Can you work these out from the drawing? Everything is in mm from the part's minimum corner. Coordinates: 2 decimals unless noted, no trailing zeros. Loops run counter-clockwise (first coordinate to the right, second up) from the corner with the lowest first, then second, coordinate; pieces in that order, holes last. Notation, with made-up numbers: M -4.5,-29 L 10.5,-29 A22 ccw 10.5,8 Z; hole C -2.75,61 d2. An arc over 180 degrees is marked long. Write each question's results on one line, items separated by ' | '.
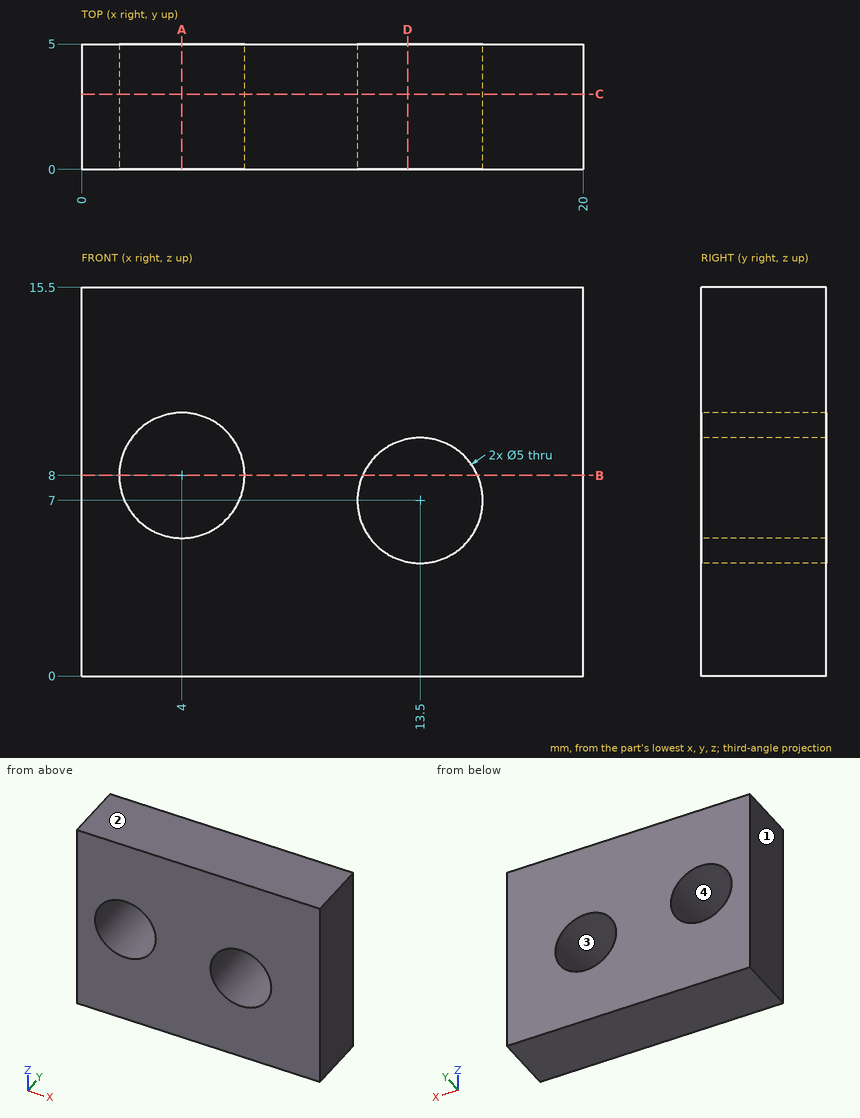
(1) Imagine slicing it at C-C, the plane y = 3. List the corners of the cut face in (x, z) for me.
Reported:
outline: M 0,0 L 20,0 L 20,15.5 L 0,15.5 Z; hole C 4,8 d5; hole C 13.5,7 d5
(2) Please list where these lines run through material, in increasing order: probe 1 along Z at (x, y) = (13.5, 3.7); probe 2 along Z at (x, y) = (4, 2.8); probe 3 along X at (y, z) = (1.5, 8.5). Write a range as from..to.
Reported:
probe 1: z = 0..4.5, 9.5..15.5 | probe 2: z = 0..5.5, 10.5..15.5 | probe 3: x = 0..1.55, 6.45..11.5, 15.5..20
(3) Will this pin go through, and if not, where does the flat tip stop? P1, Ø3, axis at x = 4, z = 8, coming from the +Y side.
Reported:
P1: passes through
(4) Imagine slicing it at B-B, the plane z = 8. List the corners of the cut face in (x, y) for me, and give its area (3 significant figures).
Reported:
outline: M 0,0 L 1.5,0 L 1.5,5 L 0,5 Z; M 6.5,0 L 11.21,0 L 11.21,5 L 6.5,5 Z; M 15.79,0 L 20,0 L 20,5 L 15.79,5 Z | area: 52.1 mm2
(5) Imagine slicing it at D-D, the plane x = 13. List the corners of the cut face in (y, z) for me, and give its area (3 significant figures).
Reported:
outline: M 0,0 L 5,0 L 5,4.55 L 0,4.55 Z; M 0,9.45 L 5,9.45 L 5,15.5 L 0,15.5 Z | area: 53.0 mm2
(6) Imagine slicing it at A-A, the plane x = 4. List the corners of the cut face in (y, z) for me.
Reported:
outline: M 0,0 L 5,0 L 5,5.5 L 0,5.5 Z; M 0,10.5 L 5,10.5 L 5,15.5 L 0,15.5 Z
(7) If we mould it in two halves opening along X, with no side actions, what happens to the marked faces 1, 2, 3 and 4? For each: released by +X, released by -X, zero draft, split by the parting line, or undercut.
Reported:
face 1: released by -X | face 2: zero draft | face 3: undercut | face 4: undercut
